Model file for the job. Use its own axes, mm. A direction names the side the tool comes from. Round coordinates to 2 decimals unless told otherwise and drop trailing zeros. Loops run counter-clockwise (first coordinate to the right, second up) from the corner with the lowest first, then second, coordinate; pieces in that order, holes last. Notation, with made-up numbers: (32, 56.5) -> (52, 56.5) arc R27 ccw to (52, 81.5) -> close; hole circle Ø3 at (18.5, 59). An arc over 180 degrees is marked (long way). Use a Markdown table: item, result.
from build123d import *

# Parameters (mm, degrees)
SKETCH1_R           = 4.318
BOSS_EXTRUDE1_DEPTH = 2.032
SKETCH2_W           = 5.0292
SKETCH2_H           = 4.318
BOSS_EXTRUDE2_DEPTH = 4.572
SKETCH3_R           = 1.651
CUT_EXTRUDE1_DEPTH  = 7.604


with BuildPart() as part:
    # Sketch1 → Boss-Extrude1 (new body)
    with BuildSketch(Plane(origin=(0, 0, 0), x_dir=(1, 0, 0), z_dir=(0, 1, 0))):
        Circle(SKETCH1_R)
    extrude(amount=BOSS_EXTRUDE1_DEPTH)

    # Sketch2 → Boss-Extrude2 (add)
    with BuildSketch(Plane(origin=(0, 2.032, 0), x_dir=(1, 0, 0), z_dir=(0, 1, 0))):
        Rectangle(SKETCH2_W, SKETCH2_H)
    extrude(amount=BOSS_EXTRUDE2_DEPTH)

    # Sketch3 → Cut-Extrude1 (cut, through all)
    with BuildSketch(Plane(origin=(0, 6.604, 0), x_dir=(1, 0, 0), z_dir=(0, 1, 0))):
        Circle(SKETCH3_R)
    extrude(amount=-CUT_EXTRUDE1_DEPTH, mode=Mode.SUBTRACT)


solid = part.part
Q1. Tool access for faces 1 (the face through (2.515, 4, 0)), 2 (the face through (-2.515, 4, 0)), 3 (the face through (0, 4, -2.159)): list every direction of +Z, -Z, +X, -X, +Y, -Y with a clear straight run to the whole face (end or side of a thin tool).
Results list:
| item | result |
|---|---|
| face 1 | +Z, -Z, +X, +Y |
| face 2 | +Z, -Z, -X, +Y |
| face 3 | -Z, +X, -X, +Y |
Q2. Band-saw the part on D-D, the plane x = -2. Give the cut face in (y, z), plus the area to 3 significant figures.
Results list:
| item | result |
|---|---|
| outline | (0, -3.83) -> (2.03, -3.83) -> (2.03, -2.16) -> (6.6, -2.16) -> (6.6, 2.16) -> (2.03, 2.16) -> (2.03, 3.83) -> (0, 3.83) -> close |
| area | 35.3 mm² |
Q3. Flat gauge pins, fed straight in: pin 1 (2 mm diameter, centred on y = 3.5, z = 0.5, fed in from +X); pin 2 (2 mm diameter, centred on y = 3.5, z = 0, fed in from -X); pin 3 (1.4 mm diameter, centred on x = 0, y = 4, fed in from +Z). Where does each tip first touch, or does it go through?
Results list:
| item | result |
|---|---|
| pin 1 | stops at x = 2.51 |
| pin 2 | stops at x = -2.51 |
| pin 3 | stops at z = 2.16 |
Q4. Band-saw the part on B-B, the plane y = 5.25. Give the cut face in (x, z), plus the area to 3 significant figures.
Results list:
| item | result |
|---|---|
| outline | (-2.51, -2.16) -> (2.51, -2.16) -> (2.51, 2.16) -> (-2.51, 2.16) -> close; hole circle Ø3.3 at (0, 0) |
| area | 13.2 mm² |
Q5. Band-saw the part on A-A, the plane z = 0. Give the cut face in (x, y).
Results list:
| item | result |
|---|---|
| outline | (-4.32, 0) -> (-1.65, 0) -> (-1.65, 6.6) -> (-2.51, 6.6) -> (-2.51, 2.03) -> (-4.32, 2.03) -> close; (1.65, 0) -> (4.32, 0) -> (4.32, 2.03) -> (2.51, 2.03) -> (2.51, 6.6) -> (1.65, 6.6) -> close |
Q6. Drill centre lines: L1, parallel to X at y = 3.75, z = 0; L2, parallel to Z at x = 0, y = 2.5; L3, parallel to X at y = 1.25, z = 0.25. Where is each one in solid material? Low to high. Write a range as from..to.
Results list:
| item | result |
|---|---|
| L1 | x = -2.51..-1.65, 1.65..2.51 |
| L2 | z = -2.16..-1.65, 1.65..2.16 |
| L3 | x = -4.31..-1.63, 1.63..4.31 |
Q7. Band-saw the part on C-C, the plane x = 0. Give the cut face in (y, z).
Results list:
| item | result |
|---|---|
| outline | (0, -4.32) -> (2.03, -4.32) -> (2.03, -2.16) -> (6.6, -2.16) -> (6.6, -1.65) -> (0, -1.65) -> close; (0, 1.65) -> (6.6, 1.65) -> (6.6, 2.16) -> (2.03, 2.16) -> (2.03, 4.32) -> (0, 4.32) -> close |
